```python
from build123d import *

# Parameters (mm, degrees)
CHAMFER1_SIZE       = 2.75
SKETCH2_OUTSIDE_W   = 12.126
SKETCH2_OUTSIDE_H   = 12.126
SKETCH2_OUTSIDE_W_2 = 5
SKETCH2_OUTSIDE_H_2 = 5
CUT_EXTRUDE1_DEPTH  = 6.8
CHAMFER2_SIZE       = 0.5


with BuildPart() as part:
    # Sketch1 → Revolve1 (revolve)
    with BuildSketch(Plane.XY, mode=Mode.PRIVATE) as revolve1_sk:
        Polygon((0, -8), (2, -8), (2, 0), (3, 0), (3, 10.8), (0, 10.8), align=None)
    revolve(revolve1_sk.sketch.rotate(Axis((0, -10.593240764, 0), (0, 1, 0)), 90), axis=Axis((0, -10.593240764, 0), (0, 1, 0)))

    # Chamfer1
    chamfer1_edges = [part.edges().sort_by_distance(p)[0] for p in [
        (0, 10.8, 3),
    ]]
    chamfer(chamfer1_edges, length=CHAMFER1_SIZE)

    # Sketch2 outside → Cut-Extrude1 (cut)
    with BuildSketch(Plane(origin=(0, 10.8, 0), x_dir=(1, 0, 0), z_dir=(0, 1, 0))):
        Rectangle(SKETCH2_OUTSIDE_W, SKETCH2_OUTSIDE_H)
        Rectangle(SKETCH2_OUTSIDE_W_2, SKETCH2_OUTSIDE_H_2, mode=Mode.SUBTRACT)
    extrude(amount=-CUT_EXTRUDE1_DEPTH, mode=Mode.SUBTRACT)

    # Chamfer2
    chamfer2_edges = [part.edges().sort_by_distance(p)[0] for p in [
        (0, -8, 2),
    ]]
    chamfer(chamfer2_edges, length=CHAMFER2_SIZE)


solid = part.part
```
Here's how the part is built. I have some questions about the finished solid (model axes, mm). A direction names the side the tool comes from. Give positions to 0.01 mm unless a question says otherwise; leave off trailing zeros. Write each loop counter-clockwise with the first axis right and the second up, starting at its lowest first coordinate (ties: lowest second). Pieces come first, ordered by that corner, then holes. Notation, with made-up numbers: (72.25, 88) -> (120.25, 88) arc R33 ccw to (120.25, 124) -> close; hole circle Ø5 at (72, 28). An arc over 180 degrees is marked (long way). Use one line per item in the form item = value.
1) Suppose I cut it at B-B (z = 0). Please give me the cut outline in (x, y).
Verdict:
outline = (-3, 0) -> (-2, 0) -> (-2, -7.5) -> (-1.5, -8) -> (1.5, -8) -> (2, -7.5) -> (2, 0) -> (3, 0) -> (3, 4) -> (2.5, 4) -> (2.5, 8.55) -> (0.25, 10.8) -> (-0.25, 10.8) -> (-2.5, 8.55) -> (-2.5, 4) -> (-3, 4) -> close
2) On a 3-axis mill with a long thin cutter (end or side, diameter ignored), from which of +Z, -Z, +X, -X, +Y, -Y can I reach the whole of each face in a straight line? I mean faces 1 (the face through (2, -4, 0)), 2 (the face through (0, 6, 2.5)), 3 (the face through (2.5, 6, 0)). Say none if no direction works.
Verdict:
face_1 = -Y
face_2 = +Z, +X, -X, +Y
face_3 = +Z, -Z, +X, +Y
3) Suppose I cut it at A-A (y = 4.25). Please give me the cut outline in (x, z).
Verdict:
outline = (-2.5, -1.66) arc R3 ccw to (-1.66, -2.5) -> (1.66, -2.5) arc R3 ccw to (2.5, -1.66) -> (2.5, 1.66) arc R3 ccw to (1.66, 2.5) -> (-1.66, 2.5) arc R3 ccw to (-2.5, 1.66) -> close
4) Suppose I cut it at D-D (y = -4.25). Please give me the cut outline in (x, z), and give its area (3 significant figures).
Verdict:
outline = circle Ø4 at (0, 0)
area = 12.6 mm2
5) If I drill on L1, parallel to X at y = -2, z = 0; L2, parallel to Y at x = 0.45, z = -2.7; L3, parallel to Z at x = -1.6, y = 7.5, over which ranges is the centre line in solid material (lowest first)? Write a range as [from, to].
Verdict:
L1 = [-2, 2]
L2 = [0, 4]
L3 = [-2.5, 2.5]
6) I'm going to push flat-ended pins straight in: pin 1 (0.6 mm diameter, centred on x = -0.5, z = -3, fed in from +Y); pin 2 (3 mm diameter, centred on x = 1.5, y = -0.5, fed in from +Z); pin 3 (0.6 mm diameter, centred on x = 2.5, z = 0, fed in from +Y); pin 4 (3 mm diameter, centred on x = -1.5, y = -5, fed in from +Z). Where does each tip first touch, or does it pass through?
Verdict:
pin_1 = 4
pin_2 = 3
pin_3 = 8.85
pin_4 = 2
7) Suppose I cut it at C-C (x = 0). Please give me the cut outline in (y, z).
Verdict:
outline = (-8, -1.5) -> (-7.5, -2) -> (0, -2) -> (0, -3) -> (4, -3) -> (4, -2.5) -> (8.55, -2.5) -> (10.8, -0.25) -> (10.8, 0.25) -> (8.55, 2.5) -> (4, 2.5) -> (4, 3) -> (0, 3) -> (0, 2) -> (-7.5, 2) -> (-8, 1.5) -> close
